Can you work these out from the drawing? Everything is in mm from the part's minimum corner. A direction names the side the tool comes from. Coordinates: 2 decimals unless noted, no trailing zeros. Order: outer loops, then holes, each group sorted by start corner. A loop starts at its lowest first (then second) coordinate and runs counter-clockwise, first axis right, second up. Notation, with made-up numbers: (-17, 22.25) - (41, 22.25) arc R15 cw to (41, 26.25) - close; hole circle Ø6 at (66, 66.5). An arc over 180 degrees is marked (long way). Use one line per item in the form item = value. Start each with the question number.
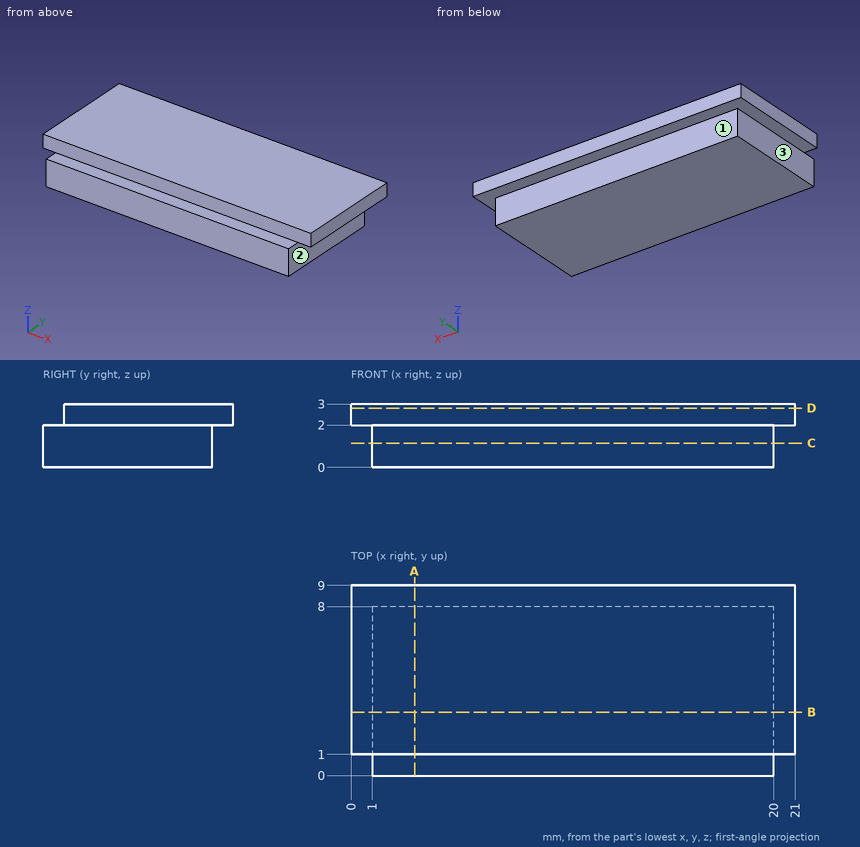
1) Suppose I cut it at A-A, the plane x = 3. List the corners of the cut face in (y, z) for me.
2) Suppose I cut it at C-C, the plane z = 1.15. List the corners of the cut face in (x, y) for me.
3) Suppose I cut it at D-D, the plane z = 2.8. List the corners of the cut face in (x, y) for me.
4) Which directions (+Z, -Z, +X, -X, +Y, -Y) give clear straight access to the entire face, cutting with the end or side of a thin tool? Please do the marked faces 1, 2 and 3.
5) For pin 1 (1 mm diameter, centred on x = 14, z = 1, fed in from +Y); pin 2 (0.6 mm diameter, centred on y = 5.5, z = 1.5, fed in from +X); pin 3 (0.8 mm diameter, centred on x = 9.5, z = 2.5, fed in from -Y), each with a flat end and sliding along its axis, tell me the tip position at first contact or that it passes through.
6) I need wall thicknesses on probe 1 along Y at (x, z) = (19.25, 1.6); probe 2 along Z at (x, y) = (1.5, 8.25); probe 3 along X at (y, z) = (5.75, 0.3). Which ranges of each line are inside material? Lowest first, please. Write a range as [from, to].
7) Suppose I cut it at B-B, the plane y = 3. List the corners of the cut face in (x, z) for me, then the cut area to 3 significant figures.
From the geometry:
q1.outline = (0, 0) - (8, 0) - (8, 2) - (9, 2) - (9, 3) - (1, 3) - (1, 2) - (0, 2) - close
q2.outline = (1, 0) - (20, 0) - (20, 8) - (1, 8) - close
q3.outline = (0, 1) - (21, 1) - (21, 9) - (0, 9) - close
q4.face_1 = -Z, +X, -X, +Y
q4.face_2 = -Z, +X, +Y, -Y
q4.face_3 = -Z, -X, +Y, -Y
q5.pin_1 = 8
q5.pin_2 = 20
q5.pin_3 = 1
q6.probe_1 = [0, 8]
q6.probe_2 = [2, 3]
q6.probe_3 = [1, 20]
q7.outline = (0, 2) - (1, 2) - (1, 0) - (20, 0) - (20, 2) - (21, 2) - (21, 3) - (0, 3) - close
q7.area = 59.0 mm2
